from build123d import *

# Parameters (mm, degrees)
SKETCH1_W                                            = 200
SKETCH1_H                                            = 100
BLOCK_STOCK_DEPTH                                    = 50
M10_TAPPED_HOLE1_D                                   = 8.5
M10_TAPPED_HOLE1_DEPTH                               = 25
M10_TAPPED_HOLE1_TIP                                 = 2.553657631
CBORE_FOR_M8_HEX_HEAD_BOLT1_D                        = 9
CBORE_FOR_M8_HEX_HEAD_BOLT1_CBORE_D                  = 18.011
CBORE_FOR_M8_HEX_HEAD_BOLT1_CBORE_DEPTH              = 5.3
POCKET_1_DEPTH                                       = 10
CSK_FOR_M10_CROSS_RECESS_FLAT_HEAD_SCREW_D           = 11
CSK_FOR_M10_CROSS_RECESS_FLAT_HEAD_SCREW_CSINK_D     = 20
CSK_FOR_M10_CROSS_RECESS_FLAT_HEAD_SCREW_CSINK_ANGLE = 90
SLOT_DEPTH                                           = 398.580729973


with BuildPart() as part:
    # Sketch1 → Block Stock (new body)
    with BuildSketch(Plane(origin=(0, 0, 0), x_dir=(1, 0, 0), z_dir=(0, 1, 0))):
        Rectangle(SKETCH1_W, SKETCH1_H)
    extrude(amount=BLOCK_STOCK_DEPTH)

    # M10 Tapped Hole1
    with Locations(Plane(origin=(100, 0, 0), x_dir=(0, 0, -1), z_dir=(1, 0, 0))):
        with Locations((15, 15)):
            Hole(M10_TAPPED_HOLE1_D / 2, depth=M10_TAPPED_HOLE1_DEPTH)
            with Locations((0, 0, -(M10_TAPPED_HOLE1_DEPTH + M10_TAPPED_HOLE1_TIP / 2))):  # 118° drill point
                Cone(0, M10_TAPPED_HOLE1_D / 2, M10_TAPPED_HOLE1_TIP, mode=Mode.SUBTRACT)

    # CBORE for M8 Hex Head Bolt1 (through all)
    with Locations(Plane(origin=(0, 50, 0), x_dir=(-1, 0, 0), z_dir=(0, 1, 0))):
        with Locations((80, 30), (-80, -30)):
            CounterBoreHole(CBORE_FOR_M8_HEX_HEAD_BOLT1_D / 2, CBORE_FOR_M8_HEX_HEAD_BOLT1_CBORE_D / 2, CBORE_FOR_M8_HEX_HEAD_BOLT1_CBORE_DEPTH)

    # Sketch2 → Pocket 1 (cut)
    with BuildSketch(Plane(origin=(0, 50, 0), x_dir=(1, 0, 0), z_dir=(0, 1, 0))):
        with BuildLine():
            Line((-87, 40), (-51.247723472, 40))
            ThreePointArc((-51.247723472, 40), (-50.934138082, 39.983565686), (-50.6239884, 39.934442802))
            Line((-50.6239884, 39.934442802), (-18.308422367, 33.065557198))
            ThreePointArc((-18.308422367, 33.065557198), (-17.998272684, 33.016434314), (-17.684687294, 33))
            Line((-17.684687294, 33), (-6, 33))
            ThreePointArc((-6, 33), (-3.878679656, 32.121320344), (-3, 30))
            Line((-3, 30), (-3, 1))
            ThreePointArc((-3, 1), (-3.878679656, -1.121320344), (-6, -2))
            Line((-6, -2), (-32, -2))
            ThreePointArc((-32, -2), (-34.121320344, -2.878679656), (-35, -5))
            Line((-35, -5), (-35, -9))
            ThreePointArc((-35, -9), (-40, -14), (-45, -9))
            Line((-45, -9), (-45, -5))
            ThreePointArc((-45, -5), (-45.878679656, -2.878679656), (-48, -2))
            Line((-48, -2), (-57, -2))
            ThreePointArc((-57, -2), (-59.121320344, -1.121320344), (-60, 1))
            Line((-60, 1), (-60, 5))
            ThreePointArc((-60, 5), (-65, 10), (-70, 5))
            Line((-70, 5), (-70, 1))
            ThreePointArc((-70, 1), (-70.878679656, -1.121320344), (-73, -2))
            Line((-73, -2), (-87, -2))
            ThreePointArc((-87, -2), (-89.121320344, -1.121320344), (-90, 1))
            Line((-90, 1), (-90, 37))
            ThreePointArc((-90, 37), (-89.121320344, 39.121320344), (-87, 40))
        make_face()
    extrude(amount=-POCKET_1_DEPTH, mode=Mode.SUBTRACT)

    # CSK for M10 Cross Recess Flat Head Screw1 (through all)
    with Locations(Plane(origin=(0, 50, 0), x_dir=(-1, 0, 0), z_dir=(0, 1, 0))):
        with Locations((-10, 30), (35, 30)):
            CounterSinkHole(CSK_FOR_M10_CROSS_RECESS_FLAT_HEAD_SCREW_D / 2, CSK_FOR_M10_CROSS_RECESS_FLAT_HEAD_SCREW_CSINK_D / 2, counter_sink_angle=CSK_FOR_M10_CROSS_RECESS_FLAT_HEAD_SCREW_CSINK_ANGLE)

    # SlotSke → Slot (cut, through all)
    with BuildSketch(Plane(origin=(218.703654527, 50, 182.375595614), x_dir=(1, 0, 0), z_dir=(0, 1, 0))):
        with BuildLine():
            Line((-149.826827264, 162.822297807), (-168.876827264, 162.822297807))
            ThreePointArc((-168.876827264, 162.822297807), (-172.242327264, 166.187797807), (-168.876827264, 169.553297807))
            Line((-168.876827264, 169.553297807), (-149.826827264, 169.553297807))
            ThreePointArc((-149.826827264, 169.553297807), (-146.461327264, 166.187797807), (-149.826827264, 162.822297807))
        make_face()
    extrude(amount=-SLOT_DEPTH, mode=Mode.SUBTRACT)


solid = part.part
CAD build for the part. Positions are in the model's coordinates, mm. A direction names the side the tool comes from. Give positions to 0.01 mm unless a question says otherwise; leave off trailing zeros. Write each loop counter-clockwise with the first axis right and the second up, starting at its lowest first coordinate (ties: lowest second). Pieces come first, ordered by that corner, then holes. Notation, with made-up numbers: (51, 71.25) -> (98, 71.25) arc R21 ccw to (98, 104.25) -> close; hole circle Ø7 at (30, -4.75). An arc over 180 degrees is marked (long way). Return JSON: item names as keys, results as strings.
Item 1: Tool access for faces 1 (the cylindrical face through (71.68, 47.39, -33.45)), 2 (the conical face through (72.89, 15.73, -14.9)), 3 (the cylindrical face through (46.462, 25.35, 16.262)): list every direction of +Z, -Z, +X, -X, +Y, -Y with a clear straight run to the whole face (end or side of a thin tool).
Answer below:
{"face 1": "+Y", "face 2": "+X", "face 3": "+Y, -Y"}
Item 2: Drop flat-ended pins along their axis: pin 1 (12 mm diameter, centred on x = 38.5, z = 24.5, fed in from -Y); pin 2 (11.5 mm diameter, centred on x = 80, z = -30, fed in from +Y); pin 3 (2 mm diameter, centred on x = -14.5, z = -19, fed in from +Y). Give the stop position or say it passes through.
Answer below:
{"pin 1": "stops at y = 0", "pin 2": "stops at y = 44.7", "pin 3": "stops at y = 40"}
Item 3: Drill centre lines: probe 1 along Z at (x, y) = (80, 32.5); probe 2 along Z at (x, y) = (-52, 41.5); probe 3 along X at (y, z) = (45, -5). Where is each one in solid material? Low to high.
Answer below:
{"probe 1": "z = -50 to -34.5, -25.5 to 50", "probe 2": "z = -50 to -40, 2 to 50", "probe 3": "x = -100 to -90, -70 to -60, -3 to 100"}
Item 4: Band-saw the part on A-A (x = 60.5). List the corners of the cut face in (y, z).
Answer below:
{"outline": "(0, -50) -> (50, -50) -> (50, 12.82) -> (0, 12.82) -> close; (0, 19.55) -> (50, 19.55) -> (50, 50) -> (0, 50) -> close"}
Item 5: Two-plate mould, pull along X, no slides. Class faces 4 (the flat face through (-100, 25, 1)), 5 (the flat face through (-12, 45, -33)), 6 (the flat face through (-1, 50, -1)), 7 (the flat face through (59, 25, 19.553)): +X half, -X half, draft (parallel to the pull), parting line (faces both ways), or undercut.
Answer below:
{"face 4": "-X half", "face 5": "undercut", "face 6": "draft", "face 7": "undercut"}
Item 6: Band-saw the part on B-B (x = -65). List the corners of the cut face in (y, z).
Answer below:
{"outline": "(0, -50) -> (50, -50) -> (50, -40) -> (40, -40) -> (40, -10) -> (50, -10) -> (50, 50) -> (0, 50) -> close"}
